```python
from build123d import *

# Parameters (mm, degrees)
SKETCH1_W               = 125
SKETCH1_H               = 110
BOSS_EXTRUDE1_DEPTH     = 11
SKETCH4_W               = 119
SKETCH4_H               = 104
CUT_EXTRUDE1_DEPTH      = 8
SKETCH6_R               = 2
CUT_EXTRUDE6_DEPTH      = 123
CUT_EXTRUDE6_DEPTH_BACK = 4
SKETCH5_R               = 2
CUT_EXTRUDE5_DEPTH      = 108
CUT_EXTRUDE5_DEPTH_BACK = 4
FILLET2_R               = 1


with BuildPart() as part:
    # Sketch1 → Boss-Extrude1 (new body)
    with BuildSketch(Plane(origin=(0, 0, 0), x_dir=(1, 0, 0), z_dir=(0, 1, 0))):
        with Locations((-139.109907121, 22.894736842)):
            Rectangle(SKETCH1_W, SKETCH1_H)
    extrude(amount=BOSS_EXTRUDE1_DEPTH)

    # Sketch4 → Cut-Extrude1 (cut)
    with BuildSketch(Plane(origin=(0, 11, 0), x_dir=(1, 0, 0), z_dir=(0, 1, 0))):
        with Locations((-139.109907121, 22.894736842)):
            Rectangle(SKETCH4_W, SKETCH4_H)
    extrude(amount=-CUT_EXTRUDE1_DEPTH, mode=Mode.SUBTRACT)

    # Sketch6 → Cut-Extrude6 (cut, two sides)
    with BuildSketch(Plane(origin=(-198.609907121, 0, 0), x_dir=(0, 0, -1), z_dir=(1, 0, 0))) as cut_extrude6_sk:
        with Locations((-2.105263158, 6.999999953)):
            Circle(SKETCH6_R)
        with Locations((22.894736842, 6.999999953)):
            Circle(SKETCH6_R)
        with Locations((47.894736842, 7)):
            Circle(SKETCH6_R)
    extrude(amount=CUT_EXTRUDE6_DEPTH, mode=Mode.SUBTRACT)
    extrude(cut_extrude6_sk.sketch, amount=-CUT_EXTRUDE6_DEPTH_BACK, mode=Mode.SUBTRACT)

    # Sketch5 → Cut-Extrude5 (cut, two sides)
    with BuildSketch(Plane.XY.offset(-74.894736842)) as cut_extrude5_sk:
        with Locations((-169.359907121, 7)):
            Circle(SKETCH5_R)
        with Locations((-140.109907121, 7)):
            Circle(SKETCH5_R)
        with Locations((-110.859907121, 7)):
            Circle(SKETCH5_R)
    extrude(amount=CUT_EXTRUDE5_DEPTH, mode=Mode.SUBTRACT)
    extrude(cut_extrude5_sk.sketch, amount=-CUT_EXTRUDE5_DEPTH_BACK, mode=Mode.SUBTRACT)

    # Fillet2
    fillet2_edges = [part.edges().sort_by_distance(p)[0] for p in [
        (-76.609907121, 11, -22.894736842),
        (-139.109907121, 11, -77.894736842),
        (-198.609907121, 11, -22.894736842),
        (-139.109907121, 11, 29.105263158),
        (-79.609907121, 11, -22.894736842),
        (-139.109907121, 11, -74.894736842),
        (-201.609907121, 11, -22.894736842),
        (-139.109907121, 11, 32.105263158),
    ]]
    fillet(fillet2_edges, radius=FILLET2_R)


solid = part.part
```
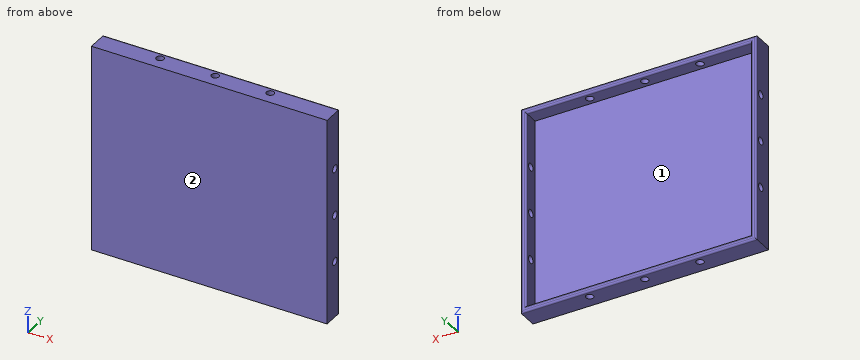
Could you check a few things on this model? Use its own coordinates, in mm. Face numbers are marked on the shaded views. Round coordinates to 2 decimals unless told otherwise and drop trailing zeros. Loops run counter-clockwise (first coordinate to the right, second up) from the corner with the lowest first, then second, coordinate; pieces in that order, holes last.
Q1. I want a section at C-C (z = 8.5). Write out the boundary of the cut face in (x, y).
Q2. Thinking about a two-plate mould opening in Z: for the marked faces 1 and 2, which applies, pulls with the +Z half, pulls with the -Z half, needs draft (parallel to the pull), parting line crosses it, or undercut?
Q3. For P1, Ø1.5, axis at x = -177.5, z = -5, coming from the +Y side, with a flat end and sliding along its axis, tell me the tip position at first contact or that it passes through.
Q4. I want a section at B-B (x = -153). Write out the boundary of the cut face in (y, z), and give its area (3 significant figures).
Q5. I want a section at D-D (y = 7). Give the number of separate pieces and of enclosed holes in the cut face, and give its area (3 significant figures).
Q6. Please list where these lines run through material, in increasing order: L1, parallel to X at y = 7, z = 30.7; L2, parallel to Z at x = -78.8, y = 7; L3, parallel to Z at x = -83, y = 6.75.
Q7. I want a section at A-A (z = -48.5). Write out the boundary of the cut face in (x, y).
Answer below:
1. outline: (-201.61, 0) - (-76.61, 0) - (-76.61, 10) arc R1 ccw to (-77.61, 11) - (-78.61, 11) arc R1 ccw to (-79.61, 10) - (-79.61, 3) - (-198.61, 3) - (-198.61, 10) arc R1 ccw to (-199.61, 11) - (-200.61, 11) arc R1 ccw to (-201.61, 10) - close
2. face 1: undercut
2. face 2: needs draft
3. P1: stops at y = 3
4. outline: (0, -77.89) - (10, -77.89) arc R1 ccw to (11, -76.89) - (11, -75.89) arc R1 ccw to (10, -74.89) - (3, -74.89) - (3, 29.11) - (10, 29.11) arc R1 ccw to (11, 30.11) - (11, 31.11) arc R1 ccw to (10, 32.11) - (0, 32.11) - close
4. area: 377 mm2
5. separate pieces: 12
5. enclosed holes: 0
5. area: 1,230 mm2
6. L1: x = -201.61 to -171.36, -167.36 to -142.11, -138.11 to -112.86, -108.86 to -76.61
6. L2: z = -77.89 to -49.89, -45.89 to -24.89, -20.89 to 0.11, 4.11 to 32.11
6. L3: z = -77.89 to -74.89, 29.11 to 32.11
7. outline: (-201.61, 0) - (-76.61, 0) - (-76.61, 5.09) - (-79.61, 5.09) - (-79.61, 3) - (-198.61, 3) - (-198.61, 5.09) - (-201.61, 5.09) - close; (-201.61, 8.91) - (-198.61, 8.91) - (-198.61, 10) arc R1 ccw to (-199.61, 11) - (-200.61, 11) arc R1 ccw to (-201.61, 10) - close; (-79.61, 8.91) - (-76.61, 8.91) - (-76.61, 10) arc R1 ccw to (-77.61, 11) - (-78.61, 11) arc R1 ccw to (-79.61, 10) - close
